```python
from build123d import *

# Parameters (mm, degrees)
SKETCH1_R           = 5
BOSS_EXTRUDE1_DEPTH = 15
SKETCH5_R           = 40
SKETCH5_R_2         = 5
BOSS_EXTRUDE2_DEPTH = 25


with BuildPart() as part:
    # Sketch1 → Boss-Extrude1 (new body)
    with BuildSketch(Plane.XY):
        with BuildLine():
            Line((0, 0), (40, 0))
            ThreePointArc((40, 0), (26.472356234, -40.750519772), (-11.908101275, -60))
            ThreePointArc((-11.908101275, -60), (-86.549117426, -40), (-11.908101275, -20))
            ThreePointArc((-11.908101275, -20), (-1.811915014, -12.466248525), (0, 0))
        make_face()
        with Locations((-46.549117426, -40)):
            Circle(SKETCH1_R, mode=Mode.SUBTRACT)
    extrude(amount=BOSS_EXTRUDE1_DEPTH)

    # Sketch5 → Boss-Extrude2 (add)
    with BuildSketch(Plane.XY.offset(15)):
        with Locations((-46.549117426, -40)):
            Circle(SKETCH5_R)
        with Locations((-46.549117426, -40)):
            Circle(SKETCH5_R_2, mode=Mode.SUBTRACT)
    extrude(amount=BOSS_EXTRUDE2_DEPTH)


solid = part.part
```
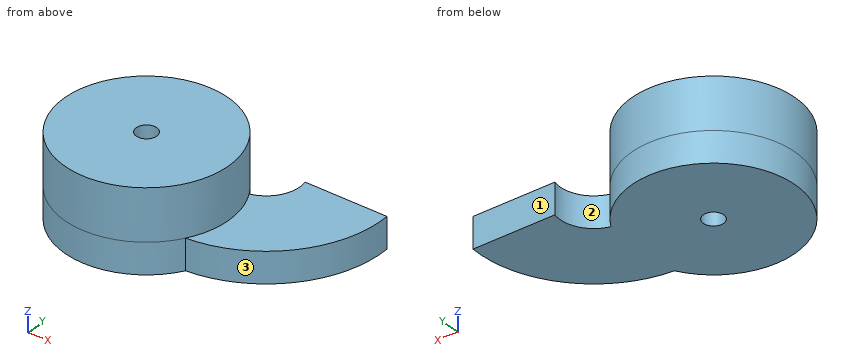
Check sheet for the modelled part. Datum: model origin and axes. Units: mm. Face numbers are marked on the shaded views. Coordinates: 2 decimals unless noted, no trailing zeros. Write each loop counter-clockwise with the first axis right and the second up, starting at its lowest first coordinate (ties: lowest second). Pieces come first, ordered by that corner, then holes. Notation, with made-up numbers: M 25.5,65 L 35.5,65 A18 cw 35.5,94 Z; hole C 21.5,-24.5 d10. An arc over 180 degrees is marked long. Write item = value, one per line. Start each with the question number.
1. Sectioned sample at B-B (z = 12). Record the cut outline in (x, y).
2. Go/stop test with flat-tipped pins: pin 1 (2 mm diameter, centred on y = -42.5, z = 26, fed in from +X); pin 2 (10 mm diameter, centred on y = -33.5, z = 7.5, fed in from -X); pin 3 (16 mm diameter, centred on x = -46.55, y = -40, fed in from +Z); pin 4 (3 mm diameter, centred on y = -58, z = 23.5, fed in from -X). Record where each tip stops, or that it passes through.
3. Sectioned sample at A-A (y = -37). Record the cut outline in (x, z), then the cut area to 3 significant figures.
4. Sectioned sample at C-C (x = -39). Record the cut outline in (y, z), then the cut area to 3 significant figures.
5. Mould release check, pull along X, two halves, no side actions. Record for the marked faces 1, 2 and 3: pulls with the +X half, pulls with the -X half, needs draft (parallel to the pull), parting line crosses it, or undercut.
6. Sectioned sample at D-D (y = -10). Record the cut outline in (x, z).
7. Thickness scan on probe 1 along X at (y, z) = (-39.5, 20); probe 2 along Z at (x, y) = (-6.5, -41); probe 3 along Y at (x, z) = (-45.5, 32). Record the ranges inside material, lowest first.
The answers:
q1.outline = M -11.91,-60 A56.1 ccw 40,0 L 0,0 A16.46 cw -11.91,-20 A40 ccw long Z; hole C -46.55,-40 d10
q2.pin_1 = -6.58
q2.pin_2 = -86.52
q2.pin_3 = 40
q2.pin_4 = -82.99
q3.outline = M -86.44,0 L -50.55,0 L -50.55,40 L -86.44,40 Z; M -42.55,0 L 29.45,0 L 29.45,15 L -6.66,15 L -6.66,40 L -42.55,40 Z
q3.area = 3,410 mm²
q4.outline = M -79.28,0 L -0.72,0 L -0.72,40 L -79.28,40 Z
q4.area = 3,140 mm²
q5.face_1 = needs draft
q5.face_2 = undercut
q5.face_3 = pulls with the +X half
q6.outline = M -73.01,0 L -20.09,0 L -20.09,40 L -73.01,40 Z; M -0.61,0 L 39.83,0 L 39.83,15 L -0.61,15 Z
q7.probe_1 = -86.55 to -51.52, -41.57 to -6.55
q7.probe_2 = 0 to 15
q7.probe_3 = -79.99 to -44.89, -35.11 to -0.01
